Geometry check sheet. Reference: drawing and pictorial views, mm from the part's lowest x, y, z. A direction names the side the tool comes from. Round coordinates to 2 decimals unless told otherwise and drop trailing zeros. Loops run counter-clockwise (first coordinate to the right, second up) from the corner with the lowest first, then second, coordinate; pieces in that order, holes last. Notation, with made-up numbers: (20.25, 45) -> (50.25, 45) arc R36 cw to (50.25, 81) -> close; hole circle Ø11 at (71, 15.5). An arc over 180 degrees is marked (long way). Use one line per item in the form item = value. Start each with the question number.
(1) Set-up check for the marked faces 1 and 2: record each of +Z, -Z, +X, -X, +Y, -Y from which the full face is reachable in a straight line by a thin tool's end or side.
(2) Sectioned sample at D-D (y = 21.75). Record the cut outline in (x, z), and give its area (3 significant figures).
(3) Draft check along X on the marked faces 3, 4, 5 and 6. Enter one of: released by +X, released by -X, zero draft, split by the parting line, or undercut.
(4) Sectioned sample at A-A (x = 12.7). Record the cut outline in (y, z) (3 decimals).
(5) Go/stop test with a flat-tipped pin: pin 1 (10 mm diameter, centred on x = 12.7, y = 12.7, fed in from +Z). Record where the tip stops, or that it passes through.
(6) Sectioned sample at C-C (z = 19.25). Record the cut outline in (x, y) (3 decimals), and give its area (3 significant figures).
(7) Material ranges on probe 1 along Y at (x, z) = (12.7, 2.75); probe 2 along Y at (x, z) = (12.7, 17.25) (3 decimals); probe 3 along Z at (x, y) = (21.5, 11.25), recorded low to high. Write a range as [from, to].
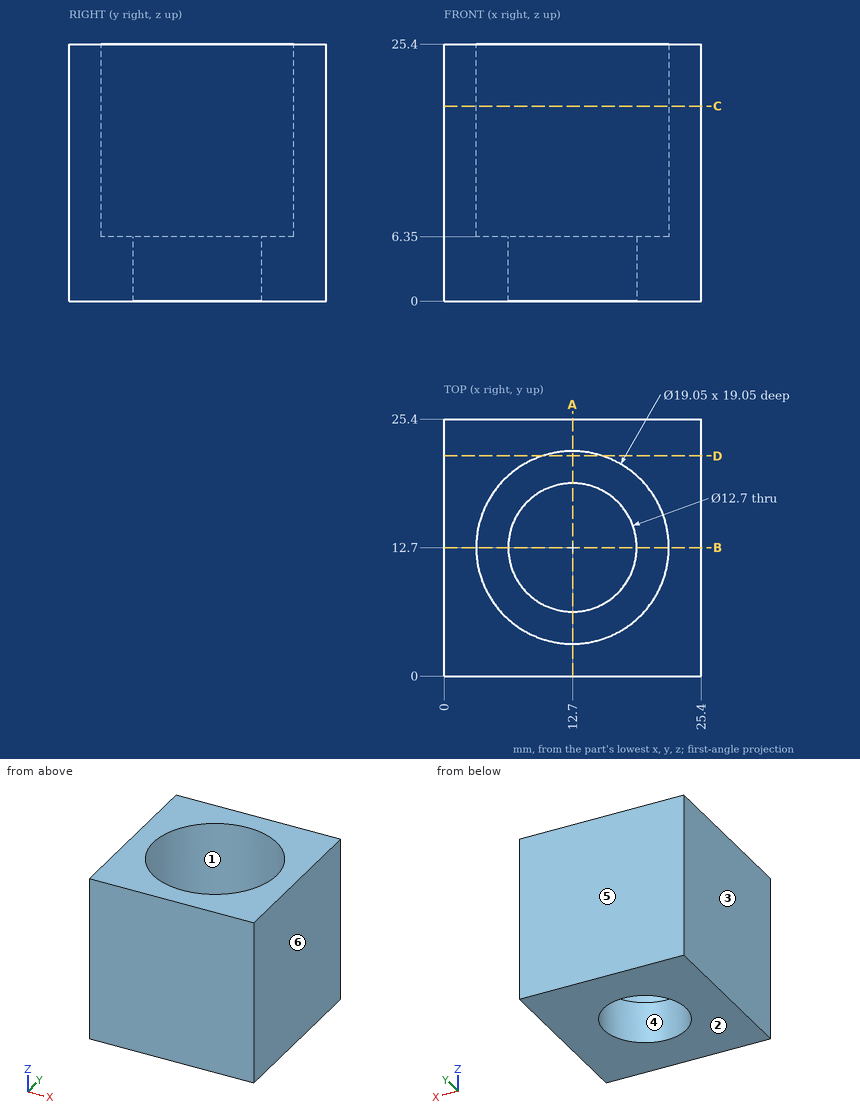
Checks:
q1.face_1 = +Z
q1.face_2 = -Z, +X, -X, +Y, -Y
q2.outline = (0, 0) -> (25.4, 0) -> (25.4, 25.4) -> (15.67, 25.4) -> (15.67, 6.35) -> (9.73, 6.35) -> (9.73, 25.4) -> (0, 25.4) -> close
q2.area = 532 mm2
q3.face_3 = released by -X
q3.face_4 = undercut
q3.face_5 = zero draft
q3.face_6 = released by +X
q4.outline = (0, 0) -> (6.35, 0) -> (6.35, 6.35) -> (3.175, 6.35) -> (3.175, 25.4) -> (0, 25.4) -> close; (19.05, 0) -> (25.4, 0) -> (25.4, 25.4) -> (22.225, 25.4) -> (22.225, 6.35) -> (19.05, 6.35) -> close
q5.pin_1 = through
q6.outline = (0, 0) -> (25.4, 0) -> (25.4, 25.4) -> (0, 25.4) -> close; hole circle Ø19.05 at (12.7, 12.7)
q6.area = 360 mm2
q7.probe_1 = [0, 6.35], [19.05, 25.4]
q7.probe_2 = [0, 3.175], [22.225, 25.4]
q7.probe_3 = [0, 6.35]
